Read the model definition and answer for the solid it produces. Units are mm, in the model's axes. Face numbers are marked on the shaded views. A direction names the side the tool comes from. Give positions to 0.01 mm unless a question says otherwise; leave off trailing zeros. Order: outer loops, then holes, each group sorted by start corner. A loop starts at its lowest first (then second) coordinate and runs counter-clockwise, first axis right, second up. Notation, with made-up numbers: (57.25, -38.75) - (65.25, -38.75) arc R29 cw to (65.25, -7.75) - close; hole circle Ø2 at (-12.5, -11.75). An arc over 180 degrees is marked (long way). Write item = value, one per line.
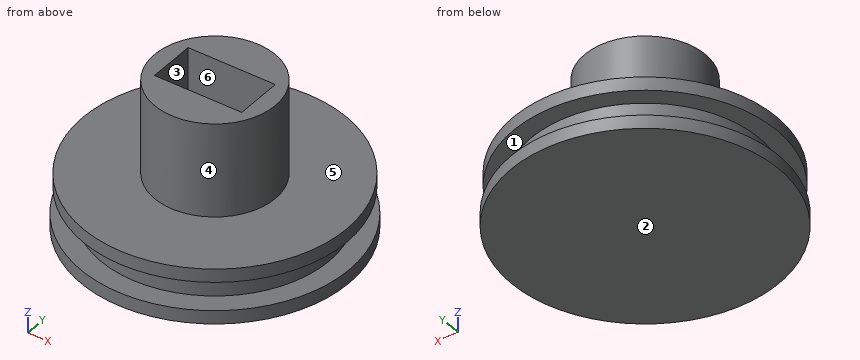
Autodesk Inventor part; units mm, degrees
ref_plane "YZ Plane" through (0, 0, 0) normal (1, 0, 0) x (0, 1, 0)
ref_plane "XZ Plane" through (0, 0, 0) normal (0, 1, 0) x (-1, 0, 0)
ref_plane "XY Plane" through (0, 0, 0) normal (0, 0, 1) x (1, 0, 0)
sketch "Sketch1" plane through (0, 0, 0) normal (0, 0, 1) x (1, 0, 0)
  circle A0 centre (0, 0) radius 10
  dimension "d0" = 20
extrude "Extrusion1" add sketch "Sketch1" along normal blind 1
sketch "Sketch2" plane through (0, 0, 1) normal (0, 0, 1) x (1, 0, 0)
  circle A0 centre (0, 0) radius 8.5
  dimension "d3" = 17
extrude "Extrusion2" add sketch "Sketch2" along normal blind 2
sketch "Sketch3" plane through (0, 0, 3) normal (0, 0, 1) x (1, 0, 0)
  circle A0 centre (0, 0) radius 9.8227
extrude "Extrusion3" add sketch "Sketch3" along normal blind 1
sketch "Sketch4" plane through (0, 0, 4) normal (0, 0, 1) x (1, 0, 0)
  circle A0 centre (0, 0) radius 4.5
  line L0 (-3.25, 1.75) -> (3.25, 1.75)
  line L1 (3.25, 1.75) -> (3.25, -1.75)
  line L2 (3.25, -1.75) -> (-3.25, -1.75)
  line L3 (-3.25, -1.75) -> (-3.25, 1.75)
  dimension "d8" = 9
  dimension "d9" = 3.5
  dimension "d10" = 6.5
  dimension "d11" = 1.75
  dimension "d12" = 3.25
extrude "Extrusion4" add sketch "Sketch4" along normal blind 7
sketch "Sketch5" plane through (0, 0, 0) normal (0, 0, -1) x (-1, 0, 0)
  point P0 (0, 0)
properties part number "Pulling Stepper Pully"
1. For the marked faces 1 and 2, determine the directions among +Z, -Z, +X, -X, +Y, -Y from which every point of the face is accessible in a straight line to the end or side of a thin tool.
Recorded:
face_1 = none
face_2 = -Z, +X, -X, +Y, -Y
2. Determine the mould class of the marked faces 3, 4, 5 and 6 for opening direction X: +X half, -X half, draft (parallel to the pull), parting line (faces both ways), or undercut.
Recorded:
face_3 = undercut
face_4 = parting line
face_5 = draft
face_6 = undercut
3. Section D-D (z = 3.25) is taken. Determine the outline of the cut face in (x, y), and give its area (3 significant figures).
Recorded:
outline = circle Ø19.65 at (0, 0)
area = 303 mm^2
4. Section A-A (x = 0) is taken. Determine the outline of the cut face in (y, z).
Recorded:
outline = (-10, 0) - (10, 0) - (10, 1) - (8.5, 1) - (8.5, 3) - (9.82, 3) - (9.82, 4) - (4.5, 4) - (4.5, 11) - (1.75, 11) - (1.75, 4) - (-1.75, 4) - (-1.75, 11) - (-4.5, 11) - (-4.5, 4) - (-9.82, 4) - (-9.82, 3) - (-8.5, 3) - (-8.5, 1) - (-10, 1) - close
5. Straight lines are drawn through the part: L1, parallel to Z at x = -8, y = -4.5; L2, parallel to Z at x = -6.25, y = -3; L3, parallel to Y at x = 0, z = 9.5. For each, find the intervals that lie inside material, in ascending order. Write a range as [from, to].
Recorded:
L1 = [0, 1], [3, 4]
L2 = [0, 4]
L3 = [-4.5, -1.75], [1.75, 4.5]
6. Section C-C (y = 0) is taken. Determine the outline of the cut face in (x, z).
Recorded:
outline = (-10, 0) - (10, 0) - (10, 1) - (8.5, 1) - (8.5, 3) - (9.82, 3) - (9.82, 4) - (4.5, 4) - (4.5, 11) - (3.25, 11) - (3.25, 4) - (-3.25, 4) - (-3.25, 11) - (-4.5, 11) - (-4.5, 4) - (-9.82, 4) - (-9.82, 3) - (-8.5, 3) - (-8.5, 1) - (-10, 1) - close
7. Section B-B (z = 10.25) is taken. Determine the outline of the cut face in (x, y), and give its area (3 significant figures).
Recorded:
outline = circle Ø9 at (0, 0); hole (-3.25, -1.75) - (3.25, -1.75) - (3.25, 1.75) - (-3.25, 1.75) - close
area = 40.9 mm^2
8. Flat-ended cylindrical pins translate along their axes: pin 1 (1 mm diameter, centred on x = 6.5, y = -6.5, fed in from -Z); pin 2 (3 mm diameter, centred on x = -0.5, z = 6, fed in from -Y); pin 3 (1 mm diameter, centred on x = -1, y = 0, fed in from +Z); pin 4 (4 mm diameter, centred on x = 2, z = 2.5, fed in from +Y). Find the tip coordinate at first contact, or state that the pin passes through.
Recorded:
pin_1 = 0
pin_2 = -4.5
pin_3 = 4
pin_4 = 9.98
